Check sheet for the drawn part. Datum: minimum x, y, z corner. Units: mm. A direction names the side the tool comes from. Round coordinates to 2 decimals unless told otherwise and drop trailing zeros. Write each loop counter-clockwise with the first axis right and the second up, starting at its lowest first coordinate (ties: lowest second). Pieces come first, ordered by that corner, then holes.
Item 1: Go/stop test with flat-tipped pins: pin 1 Ø12 at (x, z) = (8, 25) entering from -Y; pin 2 Ø1.5 at (x, y) = (3.5, 3.5) entering from -Z; pin 3 Ø1 at (y, z) = (1.5, 28.5) entering from -X; pin 4 Ø1 at (y, z) = (3, 25.5) entering from -X. Record where each tip stops, or that it passes through.
Item 2: Cross-section at A-A on y = 3.4. Enter the section's corners in (x, z), plus the area to 3 significant figures.
Item 3: Cross-section at C-C on z = 25. Enter the section's corners in (x, y), plus the area to 3 significant figures.
Item 4: Cross-section at B-B on x = 4.5. Enter the section's corners in (y, z).
Item 5: Tool access check on the marked faces 1 and 2. Record the directions out of +Z, -Z, +X, -X, +Y, -Y that give a thin tool (end or side, any length) a straight path to the whole face; none if there is none.
Item 6: Material ranges on line 1 (X direction, y = 2.05, z = 30.5); line 2 (Z direction, x = 9, y = 1.2); line 3 (Z direction, x = 27.5, y = 4.6), recorded low to high.
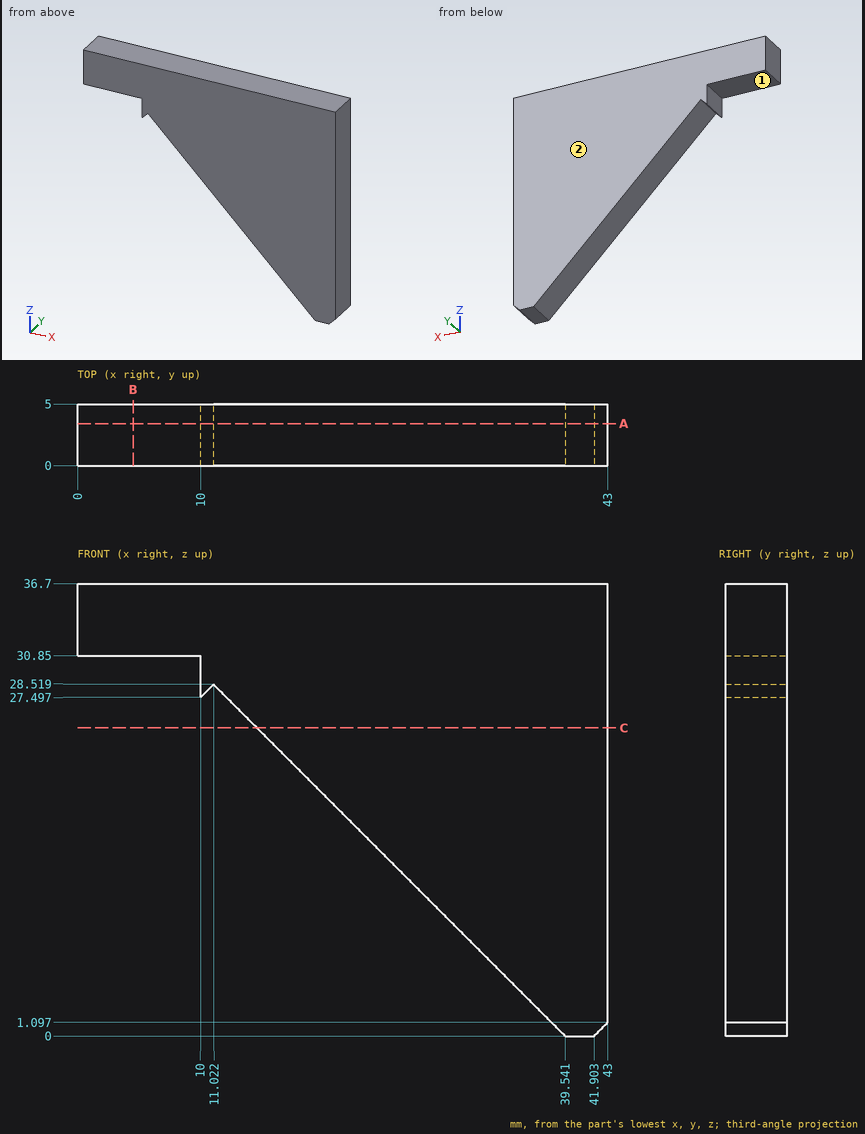
Response values:
1. pin 1: stops at y = 0
1. pin 2: stops at z = 30.85
1. pin 3: stops at x = 10
1. pin 4: stops at x = 13.54
2. outline: (0, 30.85) - (10, 30.85) - (10, 27.5) - (11.02, 28.52) - (39.54, 0) - (41.9, 0) - (43, 1.1) - (43, 36.7) - (0, 36.7) - close
2. area: 834 mm2
3. outline: (14.54, 0) - (43, 0) - (43, 5) - (14.54, 5) - close
3. area: 142 mm2
4. outline: (0, 30.85) - (5, 30.85) - (5, 36.7) - (0, 36.7) - close
5. face 1: -Z, -X, +Y, -Y
5. face 2: +Z, -Z, +X, -X, +Y
6. line 1: x = 10 to 43
6. line 2: z = 30.85 to 36.7
6. line 3: z = 12.04 to 36.7
